Can you work these out from the model? Positions are in its coordinate system, mm. Face numbers are marked on the shaded views. A direction names the side the tool comes from. Coordinates: 2 decimals unless noted, no trailing zeros. Order: outer loops, then holes, each group sorted by start corner. A loop starts at its lowest first (then second) coordinate and runs counter-clockwise, first axis right, second up.
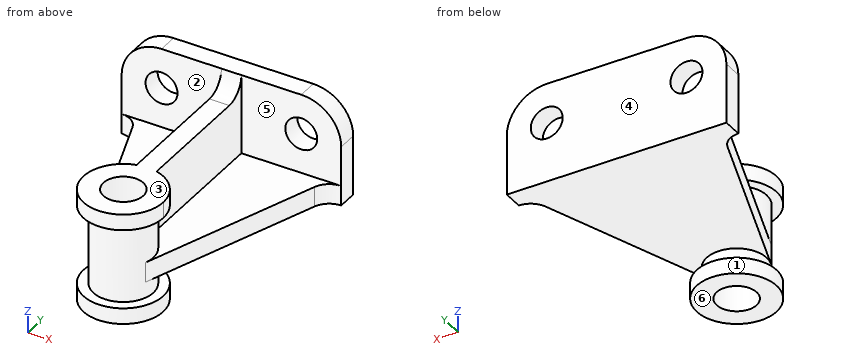
```python
from build123d import *

# Parameters (mm, degrees)
F1_DEPTH  = 10
F4_DEPTH  = 10
F6_DEPTH  = 5
F8_DEPTH  = 56
F10_DEPTH = 8
F11_R     = 20
F11_R_2   = 15
F12_DEPTH = 8
F13_R     = 10
F14_DEPTH = 56.001
F15_R     = 8
F16_DEPTH = 10


with BuildPart() as f1:
    # F0 (on Front) → F1 (new body)
    with BuildSketch(Plane.XZ):
        with BuildLine():
            Line((-55, 30), (-55, 0))
            Line((-55, 0), (55, 0))
            Line((55, 0), (55, 30))
            ThreePointArc((55, 30), (49.1421356237, 44.1421356237), (35, 50))
            Line((35, 50), (-35, 50))
            ThreePointArc((-35, 50), (-49.1421356237, 44.1421356237), (-55, 30))
        make_face()
    extrude(amount=F1_DEPTH)

    # F3 (on offset) → F4 (join)
    with BuildSketch(Plane.XY.offset(10)):
        with BuildLine():
            Line((-15.9212083525, -100), (-14.1320931815, -105.0283140623))
            ThreePointArc((-14.1320931815, -105.0283140623), (0, -115), (14.1320931815, -105.0283140623))
            Line((14.1320931815, -105.0283140623), (15.9212083525, -100))
            Line((15.9212083525, -100), (45.5786045457, -16.6477906251))
            ThreePointArc((45.5786045457, -16.6477906251), (49.2346766677, -11.8292566511), (55, -10))
            Line((55, -10), (-55, -10))
            ThreePointArc((-55, -10), (-49.2346766677, -11.8292566511), (-45.5786045457, -16.6477906251))
            Line((-45.5786045457, -16.6477906251), (-15.9212083525, -100))
        make_face()
    extrude(amount=-F4_DEPTH)

    # F5 (on Right) → F6 (join, symmetric)
    with BuildSketch(Plane.YZ):
        with BuildLine():
            Line((-100, 10), (-10, 10))
            Line((-10, 10), (-10, 40))
            Line((-10, 40), (-10, 50))
            ThreePointArc((-10, 50), (-12.9289321881, 42.9289321881), (-20, 40))
            Line((-20, 40), (-100, 40))
            Line((-100, 40), (-100, 10))
        make_face()
    extrude(amount=F6_DEPTH, both=True)

    # F7 (on face) → F8 (join)
    with BuildSketch(Plane.XY.offset(40)):
        with BuildLine():
            Line((5, -100), (5, -85.8578643763))
            ThreePointArc((5, -85.8578643763), (0, -85), (-5, -85.8578643763))
            Line((-5, -85.8578643763), (-5, -100))
            Line((-5, -100), (5, -100))
        make_face()
        with BuildLine():
            ThreePointArc((-5, -85.8578643763), (-8.6602540378, -112.2474487139), (15, -100))
            ThreePointArc((15, -100), (12.2474487139, -91.3397459622), (5, -85.8578643763))
            Line((5, -85.8578643763), (5, -100))
            Line((5, -100), (-5, -100))
            Line((-5, -100), (-5, -85.8578643763))
        make_face()
    extrude(amount=-F8_DEPTH)

    # F9 (on face) → F10 (join)
    with BuildSketch(Plane.XY.offset(40)):
        with BuildLine():
            ThreePointArc((-5, -80.635083269), (-12.2474487139, -115.8113883008), (20, -100))
            ThreePointArc((20, -100), (15.8113883008, -87.7525512861), (5, -80.635083269))
            Line((5, -80.635083269), (5, -85.8578643763))
            ThreePointArc((5, -85.8578643763), (0, -115), (-5, -85.8578643763))
            Line((-5, -85.8578643763), (-5, -80.635083269))
        make_face()
    extrude(amount=-F10_DEPTH)

    # F11 (on face) → F12 (join)
    with BuildSketch(Plane(origin=(0, 0, -16), x_dir=(1, 0, 0), z_dir=(0, 0, -1))):
        with Locations((0, 100)):
            Circle(F11_R)
        with Locations((0, 100)):
            Circle(F11_R_2, mode=Mode.SUBTRACT)
    extrude(amount=-F12_DEPTH)

    # F13 (on face) → F14 (cut, through all)
    with BuildSketch(Plane.XY.offset(40)):
        with Locations((0, -100)):
            Circle(F13_R)
    extrude(amount=-F14_DEPTH, mode=Mode.SUBTRACT)

    # F15 (on face) → F16 (cut, through all)
    with BuildSketch(Plane(origin=(0, 0, 0), x_dir=(-1, 0, 0), z_dir=(0, 1, 0))):
        with Locations((-35, 30)):
            Circle(F15_R)
        with Locations((35, 30)):
            Circle(F15_R)
    extrude(amount=-F16_DEPTH, mode=Mode.SUBTRACT)


solid = f1.part
```
1. Please list where these lines run through material, in increasing order: probe 1 along Y at (x, z) = (0, 26); probe 2 along Z at (x, y) = (35, -6.25); probe 3 along X at (y, z) = (-8.5, 33).
Completed:
probe 1: y = -115 to -110, -90 to 0
probe 2: z = 0 to 22, 38 to 50
probe 3: x = -54.77 to -42.42, -27.58 to 27.58, 42.42 to 54.77
2. Thinking about a two-plate mould opening in Y: for the marked faces 4, 5 and 6, which applies, pulls with the +Y half, pulls with the -Y half, needs draft (parallel to the pull), parting line crosses it, or undercut?
Completed:
face 4: pulls with the +Y half
face 5: undercut
face 6: needs draft
3. Imagine slicing it at B-B on z = 25. Please give me the cut outline in (x, y) (3 decimals), then the cut area to 3 significant figures.
Completed:
outline: (-55, -10) - (-41.245, -10) - (-41.245, 0) - (-55, 0) - close; (-28.755, -10) - (-5, -10) - (-5, -85.858) arc R15 ccw (long way) to (5, -85.858) - (5, -10) - (28.755, -10) - (28.755, 0) - (-28.755, 0) - close; (41.245, -10) - (55, -10) - (55, 0) - (41.245, 0) - close; hole circle Ø20 at (0, -100)
area: 2,000 mm2
4. On a 3-axis mill with a long thin cutter (end or side, diameter ignored), from which of +Z, -Z, +X, -X, +Y, -Y can I reach the whole of each face in a straight line? I mean the marked faces 1, 2 and 3. Say none if no direction works.
Completed:
face 1: -Z
face 2: +Z, -X
face 3: +Z, +X, -X, -Y
5. I'm going to push flat-ended pins straight in: pin 1 (20 mm diameter, centred on y = -49, z = 27, fed in from +X); pin 2 (18.5 mm diameter, centred on x = 35, z = 30, fed in from -Y); pin 3 (1.5 mm diameter, centred on y = -86.5, z = 27, fed in from +X); pin 4 (16 mm diameter, centred on x = 0, y = -100, fed in from +Z). Where does each tip first touch, or does it pass through?
Completed:
pin 1: stops at x = 5
pin 2: stops at y = -10
pin 3: stops at x = 7.9
pin 4: passes through
6. Imagine slicing it at D-D on x = -40. Please give me the cut outline in (y, z) (3 decimals).
Completed:
outline: (-32.326, 0) - (0, 0) - (0, 23.755) - (-10, 23.755) - (-10, 10) - (-32.326, 10) - close; (-10, 36.245) - (0, 36.245) - (0, 49.365) - (-10, 49.365) - close
7. Imagine slicing it at C-C on y = -30. Please give me the cut outline in (x, z).
Completed:
outline: (-40.83, 0) - (40.83, 0) - (40.83, 10) - (5, 10) - (5, 40) - (-5, 40) - (-5, 10) - (-40.83, 10) - close
8. Imagine slicing it at A-A on x = 0. Please give me the cut outline in (y, z), then the cut area to 3 significant figures.
Completed:
outline: (-120, -16) - (-110, -16) - (-110, 40) - (-120, 40) - (-120, 32) - (-115, 32) - (-115, -8) - (-120, -8) - close; (-90, -16) - (-80, -16) - (-80, -8) - (-85, -8) - (-85, 0) - (0, 0) - (0, 50) - (-10, 50) arc R10 cw to (-20, 40) - (-90, 40) - close
area: 4,200 mm2
